Part model, mm, in its own coordinate system. Face numbers are marked on the shaded views. A direction names the side the tool comes from. Coordinates: 2 decimals unless noted, no trailing zeros. Write each loop counter-clockwise with the first axis right and the second up, starting at its lowest first coordinate (ties: lowest second). Pieces come first, ordered by that corner, then holes. Notation, with made-up numbers: (-1, 89) -> (48, 89) arc R5 ccw to (48, 95) -> close; hole circle Ø3 at (-16.5, 31.25). An arc over 180 degrees is marked (long way). Write item = value, one per line. Start each with the question number.
Q1. Tool access for the marked faces 4, 5 and 6: list every direction of +Z, -Z, +X, -X, +Y, -Y with a clear straight run to the whole face (end or side of a thin tool).
Q2. Probe line 1 (Z direction, x = 8, y = 41); line 2 (Z direction, x = 12, y = 41); line 3 (Y direction, x = -114, z = -107.5). List the from-to ranges inside material, lowest first.
Q3. Band-saw the part on A-A, the plane y = -40. List the corners of the cut face in (x, z), plus the area to 3 significant figures.
Q4. Band-saw the part on C-C, the plane z = -41.5. List the corners of the cut face in (x, y), plus the area to 3 significant figures.
Q5. Band-saw the part on D-D, the plane y = -139. List the corners of the cut face in (x, z), plus the area to 3 significant figures.
Q6. Pin check, flat tips, straight feed: P1, Ø5, axis at y = 41, z = -123.5, coming from the +X side; P2, Ø4, axis at x = -49.5, y = -96, coming from the +Z side; P3, Ø1, axis at x = -99, y = -18.5, coming from the -Z side; P4, Ø1, axis at x = 63.5, z = -6, coming from the -Y side. Stop position of each tip, or through.
Q7. Pull direction Y, two halves, no side cores. Call the marked faces 1, 2 and 3: released by +Y, released by -Y, zero draft, split by the parting line, or undercut.
Q8. Band-saw the part on B-B, the plane x = 34. List the corners of the cut face in (y, z).
from build123d import *

# Parameters (mm, degrees)
SZKIC1_W                        = 240
SZKIC1_H                        = 240
DODANIE_WYCI_GNI_CIE1_DEPTH     = 8
SZKIC2_W                        = 240
SZKIC2_H                        = 240
SZKIC2_W_2                      = 232
SZKIC2_H_2                      = 232
DODANIE_WYCI_GNI_CIE2_DEPTH     = 50
DODANIE_WYCI_GNI_CIE6_DEPTH     = 50
ZAOKR_GLENIE1_R                 = 5
SZYK_KO_OWY1_COUNT              = 4
ZAOKR_GLENIE1_OF_SZYK_KO_OWY1_R = 5
SZKIC12_W                       = 19
SZKIC12_H                       = 28
WYTNIJ_WYCI_GNI_CIE3_DEPTH      = 275.525044395
DODANIE_WYCI_GNI_CIE7_DEPTH     = 10
SZKIC16_R                       = 2.5
WYTNIJ_WYCI_GNI_CIE4_DEPTH      = 196.842411137
SZKIC5_W                        = 10
SZKIC5_H                        = 240
DODANIE_WYCI_GNI_CIE3_DEPTH     = 21
SZKIC6_W                        = 28
SZKIC6_H                        = 240
DODANIE_WYCI_GNI_CIE4_DEPTH     = 10
SFAZOWANIE2_SIZE                = 31
WYTNIJ_WYCI_GNI_CIE2_DEPTH      = 319.144010562
WYTNIJ_WYCI_GNI_CIE2_DEPTH_BACK = 319.144010562
SZKIC9_W                        = 150
SZKIC9_H                        = 155.854455748
SZKIC10_W                       = 45
SZKIC10_H                       = 10
DODANIE_WYCI_GNI_CIE5_DEPTH     = 4.8


with BuildPart() as part:
    # Szkic1 → Dodanie-wyciągnięcie1 (new body)
    with BuildSketch(Plane(origin=(0, 0, 0), x_dir=(1, 0, 0), z_dir=(0, 1, 0))):
        Rectangle(SZKIC1_W, SZKIC1_H)
    extrude(amount=DODANIE_WYCI_GNI_CIE1_DEPTH)

    # Szkic2 → Dodanie-wyciągnięcie2 (add)
    with BuildSketch(Plane(origin=(0, 8, 0), x_dir=(1, 0, 0), z_dir=(0, 1, 0))):
        Rectangle(SZKIC2_W, SZKIC2_H)
        Rectangle(SZKIC2_W_2, SZKIC2_H_2, mode=Mode.SUBTRACT)
    extrude(amount=DODANIE_WYCI_GNI_CIE2_DEPTH)

    # Szkic11 → Dodanie-wyciągnięcie6 (add)
    with BuildSketch(Plane(origin=(0, 8, 0), x_dir=(1, 0, 0), z_dir=(0, 1, 0))):
        Polygon((-116, 116), (-66, 116), (-83.67766953, 98.32233047), (-94.284271247, 108.928932188), (-108.928932188, 94.284271247), (-98.32233047, 83.67766953), (-116, 66), align=None)
    dodanie_wyci_gni_cie6 = extrude(amount=DODANIE_WYCI_GNI_CIE6_DEPTH)

    # Zaokrąglenie1
    zaokr_glenie1_edges = [part.edges().sort_by_distance(p)[0] for p in [
        (-98.32233047, 33, -83.67766953),
        (-108.928932188, 33, -94.284271247),
        (-94.284271247, 33, -108.928932188),
        (-83.67766953, 33, -98.32233047),
    ]]
    fillet(zaokr_glenie1_edges, radius=ZAOKR_GLENIE1_R)

    # Szyk kołowy1: Dodanie-wyciągnięcie6 ×4 about axis
    szyk_ko_owy1_axis = Axis((0, 0, 0), (0, 1, 0))
    for i in range(1, SZYK_KO_OWY1_COUNT):
        add(dodanie_wyci_gni_cie6.rotate(szyk_ko_owy1_axis, i * 360 / SZYK_KO_OWY1_COUNT))

    # Zaokrąglenie1 of Szyk kołowy1
    zaokr_glenie1_of_szyk_ko_owy1_edges = [part.edges().sort_by_distance(p)[0] for p in [
        (-83.67766953, 33, 98.32233047),
        (-94.284271247, 33, 108.928932188),
        (-108.928932188, 33, 94.284271247),
        (-98.32233047, 33, 83.67766953),
        (98.32233047, 33, 83.67766953),
        (108.928932188, 33, 94.284271247),
        (94.284271247, 33, 108.928932188),
        (83.67766953, 33, 98.32233047),
        (83.67766953, 33, -98.32233047),
        (94.284271247, 33, -108.928932188),
        (108.928932188, 33, -94.284271247),
        (98.32233047, 33, -83.67766953),
    ]]
    fillet(zaokr_glenie1_of_szyk_ko_owy1_edges, radius=ZAOKR_GLENIE1_OF_SZYK_KO_OWY1_R)

    # Szkic12 → Wytnij-wyciągnięcie3 (cut, through all)
    with BuildSketch(Plane(origin=(0, 0, -120), x_dir=(-1, 0, 0), z_dir=(0, 0, -1))):
        with Locations((0, 32)):
            Rectangle(SZKIC12_W, SZKIC12_H)
    extrude(amount=-WYTNIJ_WYCI_GNI_CIE3_DEPTH, mode=Mode.SUBTRACT)

    # Szkic15 → Dodanie-wyciągnięcie7 (add)
    with BuildSketch(Plane.XY.offset(120)):
        Polygon((9.5, 45.9), (14.5, 45.9), (14.5, 35.9), (9.5, 35.9), (5.5, 35.9), (5.5, 45.9), align=None)
        Polygon((-14.5, 45.9), (-14.5, 35.9), (-9.5, 35.9), (-5.5, 35.9), (-5.5, 45.9), (-9.5, 45.9), align=None)
    dodanie_wyci_gni_cie7 = extrude(amount=DODANIE_WYCI_GNI_CIE7_DEPTH)

    # Szkic16 → Wytnij-wyciągnięcie4 (cut, through all)
    with BuildSketch(Plane(origin=(14.5, 0, 0), x_dir=(0, 0, -1), z_dir=(1, 0, 0))):
        with Locations(Location((-125, 41, 0), (0, 0, 90))):
            Circle(SZKIC16_R)
    wytnij_wyci_gni_cie4 = extrude(amount=-WYTNIJ_WYCI_GNI_CIE4_DEPTH, mode=Mode.SUBTRACT)

    # Lustro1: Dodanie-wyciągnięcie7, Wytnij-wyciągnięcie4 across plane
    add(dodanie_wyci_gni_cie7.mirror(Plane.XY))
    add(wytnij_wyci_gni_cie4.mirror(Plane.XY), mode=Mode.SUBTRACT)

    # Szkic5 → Dodanie-wyciągnięcie3 (add)
    with BuildSketch(Plane.XZ):
        with Locations((-97, 0)):
            Rectangle(SZKIC5_W, SZKIC5_H)
    extrude(amount=DODANIE_WYCI_GNI_CIE3_DEPTH)

    # Szkic6 → Dodanie-wyciągnięcie4 (add)
    with BuildSketch(Plane.XZ.offset(21)):
        with Locations((-106, 0)):
            Rectangle(SZKIC6_W, SZKIC6_H)
    extrude(amount=DODANIE_WYCI_GNI_CIE4_DEPTH)

    # Sfazowanie2
    sfazowanie2_edges = [part.edges().sort_by_distance(p)[0] for p in [
        (-92, 0, 0),
    ]]
    chamfer(sfazowanie2_edges, length=SFAZOWANIE2_SIZE - 0.0001)  # a hair under: the kernel refuses the full size

    # Szkic8 → Wyciągnięcie po profilach1 section 0
    with BuildSketch(Plane.ZY.offset(125)):
        with BuildLine():
            Line((-120, -155.854455748), (120, -155.854455748))
            Line((120, -155.854455748), (120, -145.854455748))
            Line((120, -145.854455748), (-120, -145.854455748))
            Line((-120, -145.854455748), (-120, -155.854455748))
        make_face()
    # Szkic7 → Wyciągnięcie po profilach1 section 1
    with BuildSketch(Plane.XZ):
        with BuildLine():
            Line((120, 120), (110, 120))
            Line((110, 120), (110, -120))
            Line((110, -120), (120, -120))
            Line((120, -120), (120, 120))
        make_face()
    loft()

    # Szkic9 → Wytnij-wyciągnięcie2 (cut, two sides: drawn at the far end of the back side and taken through both)
    with BuildSketch(Plane(origin=(120, 0, 0), x_dir=(0, 0, -1), z_dir=(1, 0, 0)).offset(-WYTNIJ_WYCI_GNI_CIE2_DEPTH_BACK)):
        with Locations((0, -77.927227874)):
            Rectangle(SZKIC9_W, SZKIC9_H)
    extrude(amount=WYTNIJ_WYCI_GNI_CIE2_DEPTH + WYTNIJ_WYCI_GNI_CIE2_DEPTH_BACK, mode=Mode.SUBTRACT)

    # Szkic10 → Dodanie-wyciągnięcie5 (add)
    with BuildSketch(Plane.ZY.offset(125)):
        with Locations((97.5, -150.854455748)):
            Rectangle(SZKIC10_W, SZKIC10_H)
        with Locations((-97.5, -150.854455748)):
            Rectangle(SZKIC10_W, SZKIC10_H)
    extrude(amount=DODANIE_WYCI_GNI_CIE5_DEPTH)


solid = part.part
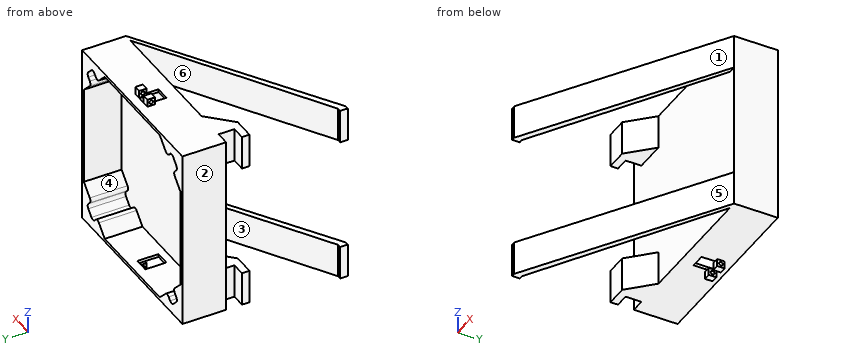
Ans:
q1.face_4 = +Y
q1.face_5 = +Z, -Z, +X, -Y
q1.face_6 = +Z, -Z
q2.line_1 = -130 to -127.5, -122.5 to -120, 120 to 122.5, 127.5 to 130
q2.line_2 = -130 to -127.5, -122.5 to -116, 116 to 122.5, 127.5 to 130
q2.line_3 = -148.86 to -139.03, -31 to -21, 0 to 58
q3.outline = (45.55, -120) -> (57.12, -120) -> (57.12, -75) -> (45.55, -75) -> close; (45.55, 75) -> (57.12, 75) -> (57.12, 120) -> (45.55, 120) -> close
q3.area = 1,040 mm2
q4.outline = (-120, 0) -> (120, 0) -> (120, 58) -> (116, 58) -> (116, 8) -> (-116, 8) -> (-116, 58) -> (-120, 58) -> close
q4.area = 2,320 mm2
q5.outline = (-113.96, -120) -> (-98.51, -120) -> (-98.51, -75) -> (-113.96, -75) -> close; (-113.96, 75) -> (-98.51, 75) -> (-98.51, 120) -> (-113.96, 120) -> close
q5.area = 1,390 mm2
q6.P1 = 14.5
q6.P2 = through
q6.P3 = -120
q6.P4 = 0
q7.face_1 = released by -Y
q7.face_2 = zero draft
q7.face_3 = undercut
q8.outline = (-54.71, -120) -> (-47.17, -120) -> (-47.17, -75) -> (-54.71, -75) -> close; (-54.71, 75) -> (-47.17, 75) -> (-47.17, 120) -> (-54.71, 120) -> close; (0, -120) -> (58, -120) -> (58, -116) -> (8, -116) -> (8, 116) -> (58, 116) -> (58, 120) -> (0, 120) -> close
